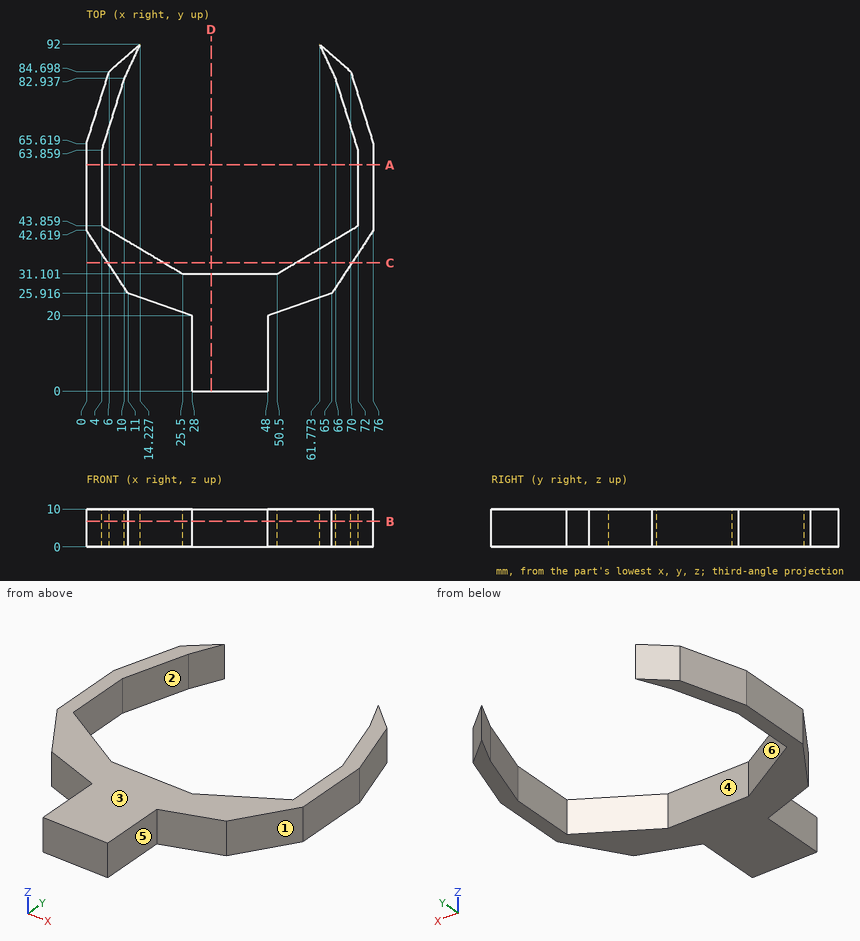
Geometry: see drawing. Coordinates: mm, zero at the bounding-box minimum. A direction names the side the tool comes from. Give positions to 0.01 mm unless a question says otherwise; leave off trailing zeros. Loops run counter-clockwise (first coordinate to the right, second up) from the corner with the lowest first, then second, coordinate; pieces in that order, holes last. Notation, with made-up numbers: (55, 39) -> (77, 39) arc R22 ccw to (77, 49) -> close; hole circle Ø8 at (-34.5, 15). An arc over 180 degrees is marked (long way). Use one line per item in the form item = value.
Item 1: Line query: probe 1 along X at (y, z) = (52, 3.75); probe 2 along X at (y, z) = (36.5, 0.5) (1 decimal); probe 3 along Y at (x, z) = (31.5, 2.75). Output: solid intervals per line, ascending.
A:
probe_1 = 0 to 4, 72 to 76
probe_2 = 4 to 16.4, 59.6 to 72
probe_3 = 0 to 31.1
Item 2: Section query C-C on y = 34. Output: boundary loops of the cut face in (x, z) (1 decimal), and give its area (3 significant figures).
A:
outline = (5.7, 0) -> (20.6, 0) -> (20.6, 10) -> (5.7, 10) -> close; (55.4, 0) -> (70.3, 0) -> (70.3, 10) -> (55.4, 10) -> close
area = 299 mm^2
Item 3: Access query for the marked faces 4, 5 and 6. Directions: +Z, -Z, +X, -X, +Y, -Y. A direction counts if a zero-diameter tool reaches every point of the face in a straight line with its end or side. Return the directions, or none.
A:
face_4 = +Z, -Z, +Y
face_5 = +Z, -Z, +X, -Y
face_6 = +Z, -Z
Item 4: Section query B-B on z = 6.75. Output: boundary loops of the cut face in (x, y).
A:
outline = (0, 42.62) -> (11, 25.92) -> (28, 20) -> (28, 0) -> (48, 0) -> (48, 20) -> (65, 25.92) -> (76, 42.62) -> (76, 65.62) -> (70, 84.7) -> (61.77, 92) -> (66, 82.94) -> (72, 63.86) -> (72, 43.86) -> (50.5, 31.1) -> (25.5, 31.1) -> (4, 43.86) -> (4, 63.86) -> (10, 82.94) -> (14.23, 92) -> (6, 84.7) -> (0, 65.62) -> close
Item 5: Pin query (flat end, axial travel): P1, Ø3, axis at x = 43, z = 6, coming from the +Y side; P2, Ø1, axis at y = 53, z = 7.5, coming from the -X side; P3, Ø4, axis at x = 58.5, z = 4, coming from the +Y side (1 decimal); P4, Ø3, axis at y = 14, z = 7.5, coming from the +X side. Return the tip coordinate at first contact, or that it passes through.
A:
P1 = 31.1
P2 = 0
P3 = 37
P4 = 48
Item 6: Section query D-D on x = 33. Output: boundary loops of the cut face in (y, z).
A:
outline = (0, 0) -> (31.1, 0) -> (31.1, 10) -> (0, 10) -> close
Item 7: Section query A-A on y = 60. Output: boundary loops of the cut face in (x, z).
A:
outline = (0, 0) -> (4, 0) -> (4, 10) -> (0, 10) -> close; (72, 0) -> (76, 0) -> (76, 10) -> (72, 10) -> close
Item 8: Draft query along X for the marked faces 1, 2 and 3. Return one class per face: pulls with the +X half, pulls with the -X half, needs draft (parallel to the pull), parting line crosses it, or undercut.
A:
face_1 = pulls with the +X half
face_2 = undercut
face_3 = needs draft
